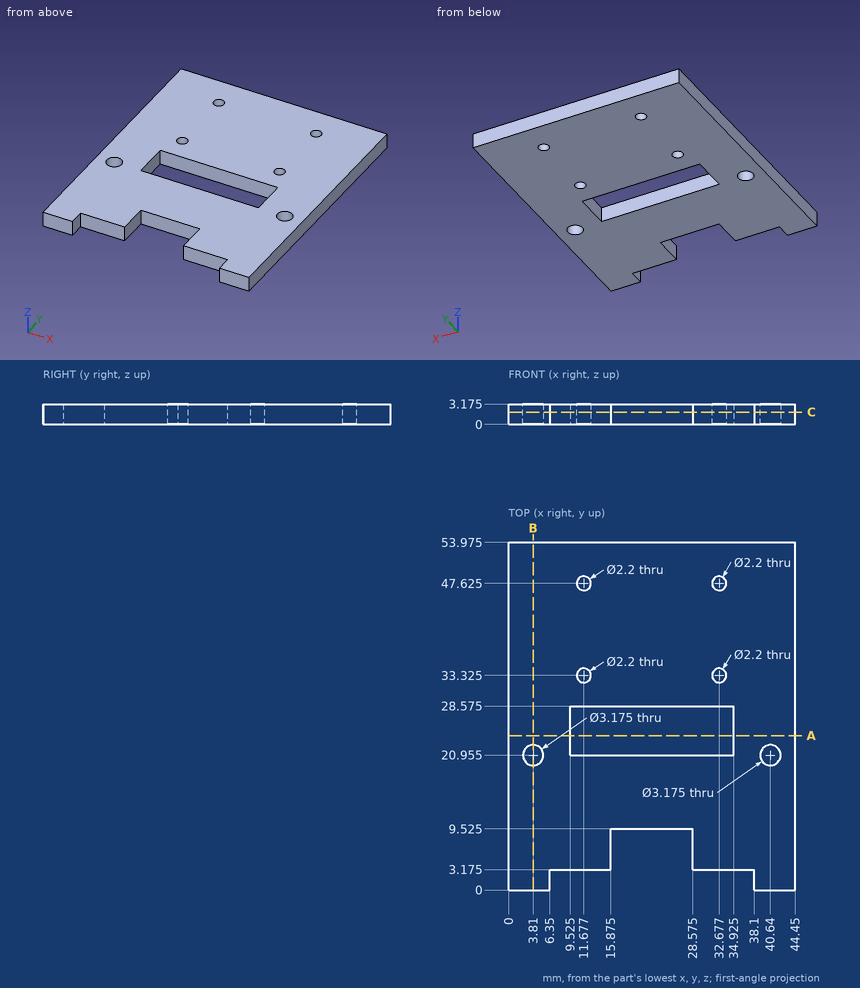
For this review, use the dimensioned drawing (mm, ordinates from the lowest corner) and the shaded views. Round coordinates to 2 decimals unless told otherwise and drop trailing zeros. Write each loop counter-clockwise with the first axis right and the second up, starting at its lowest first coordinate (ties: lowest second). Pieces come first, ordered by that corner, then holes. Notation, with made-up numbers: M 26,-10.75 L 59,-10.75 A23 cw 59,9.25 Z; hole C 11,17.5 d10. An arc over 180 degrees is marked long. Use CSV: the item, a comma, the result in double quotes. Start each with the question number.
(1) We need section A-A, the plane y = 24. State the section outline as (x, z) points (3 decimals), then the cut area to 3 significant figures.
(2) For line 1 along X through (y, z) = (26.5, 3) (3 decimals); line 2 along Y through (x, z) = (22, 3) (3 decimals); line 3 along Y through (x, z) = (40.64, 1.6) (1 decimal), list the stretches that pass through material, from the lowest coordinate up.
(3) We need section C-C, the plane z = 1.9. State how many separate pieces and enclosed holes the cut face has, then the cut area to 3 significant figures.
(4) Clearance check with flat-ended pins moving along their axes: P1, Ø1.6, axis at x = 20, z = 1.5, coming from the -Y side (3 decimals); P2, Ø1.6, axis at x = 33.5, z = 1, coming from the -Y side (3 decimals). State where each tip first meets the part, or that it passes through.
(5) We need section B-B, the plane x = 3.81. State the section outline as (y, z) points (1 decimal), then the cut area to 3 significant figures.
Findings:
1,outline,"M 0,0 L 9.525,0 L 9.525,3.175 L 0,3.175 Z; M 34.925,0 L 44.45,0 L 44.45,3.175 L 34.925,3.175 Z"
1,area,"60.5 mm^2"
2,line 1,"0 to 9.525, 34.925 to 44.45"
2,line 2,"9.525 to 20.955, 28.575 to 53.975"
2,line 3,"0 to 19.4, 22.5 to 54"
3,separate pieces,"1"
3,enclosed holes,"7"
3,area,"1,990 mm^2"
4,P1,"y = 9.525"
4,P2,"y = 3.175"
5,outline,"M 0,0 L 19.4,0 L 19.4,3.2 L 0,3.2 Z; M 22.5,0 L 54,0 L 54,3.2 L 22.5,3.2 Z"
5,area,"161 mm^2"
